Verification items for the finished model (mm, model axes). Face numbers are marked on the shaded views. A direction names the side the tool comes from. Coordinates: 2 decimals unless noted, no trailing zeros. Write each loop counter-clockwise with the first axis right and the second up, starting at its lowest first coordinate (ties: lowest second). Pieces come first, ordered by that corner, then holes. Notation, with made-up numbers: (-30.75, 64.5) - (8.25, 64.5) arc R14 ccw to (8.25, 76.5) - close; hole circle Ø5 at (-4, 14). An arc over 180 degrees is marked (long way). Use one line per item in the form item = value. Start each with the question number.
(1) Gauge pin test, flat ends, axial feed: pin 1 Ø4 at (y, z) = (6.125, -23.275) entering from -X; pin 2 Ø12 at (x, y) = (13.5, 11) entering from +Z; pin 3 Ø3.5 at (x, z) = (5, -25) entering from -Y; pin 4 Ø4 at (x, y) = (-1.5, 22.5) entering from +Z. Record the tip position at first contact, or that the pin passes through.
(2) Material ranges on line 1 (X direction, y = 73.4, z = -38.4); line 2 (X direction, y = 7, z = -18); line 3 (Z direction, x = 11, y = 31), recorded low to high. Write a range as [from, to].
(3) Sectioned sample at D-D (z = -8). Record the cut outline in (x, y).
(4) Sectioned sample at B-B (x = 7). Record the cut outline in (y, z).
(5) Tool access check on the marked faces 1, 2 and 3. Record the directions out of +Z, -Z, +X, -X, +Y, -Y that give a thin tool (end or side, any length) a straight path to the whole face; none if there is none.
(6) Sectioned sample at A-A (z = -38.4). Record the cut outline in (x, y).
(7) Sectioned sample at C-C (y = 29). Record the cut outline in (x, z), and give its area (3 significant figures).
Autodesk Inventor part; units mm, degrees
ref_plane "YZ Plane" through (0, 0, 0) normal (1, 0, 0) x (0, 1, 0)
ref_plane "XZ Plane" through (0, 0, 0) normal (0, 1, 0) x (-1, 0, 0)
ref_plane "XY Plane" through (0, 0, 0) normal (0, 0, 1) x (1, 0, 0)
sketch "Sketch1" plane through (0, 0, 0) normal (0, 1, 0) x (-1, 0, 0)
  line L0 (16.9826, -9.4) -> (-20.8174, -9.4)
  line L1 (-20.8174, -9.4) -> (-20.8174, -29.4)
  line L2 (-20.8174, -29.4) -> (16.9826, -29.4)
  line L3 (16.9826, -29.4) -> (16.9826, -9.4)
  line L4 (7.0826, -29.4) -> (-10.9174, -29.4)
  line L5 (-10.9174, -29.4) -> (-10.9174, -17.15)
  line L6 (-10.9174, -17.15) -> (7.0826, -17.15)
  line L7 (7.0826, -17.15) -> (7.0826, -29.4)
  point P0 (0, 0)
  dimension "d0" = 37.8
  dimension "d1" = 20
  dimension "d2" = 9.9
  dimension "d3" = 9.9
  dimension "d4" = 12.25
extrude "Extrusion1" add sketch "Sketch1" along normal blind 76.05
extrude "Extrusion2" cut sketch "Sketch1" along normal blind 12.25 contours L2 L5 L6 L7
sketch "Sketch2" plane through (0, 0, 0) normal (0, -1, 0) x (1, 0, 0)
  line L0 (-16.9826, -29.4) -> (-16.9826, -9.4)
  line L1 (-16.9826, -9.4) -> (20.8174, -9.4)
  line L2 (20.8174, -9.4) -> (20.8174, 0.6)
  line L3 (20.8174, 0.6) -> (-16.9826, 0.6)
  line L4 (-16.9826, 0.6) -> (-16.9826, -9.4)
  point P0 (0, 0)
  dimension "d10" = 10
extrude "Extrusion3" add sketch "Sketch2" against normal blind 20
sketch "Sketch4" plane through (20.8174, 0, -29.4) normal (1, 0, 0) x (0, 0, -1)
  line L0 (0, 0) -> (-30, 0)
  line L1 (-30, 0) -> (-30, 20)
  line L2 (-30, 0) -> (-30, 20)
  line L3 (-30, 20) -> (-20, 20)
  line L4 (-30, 0) -> (-30, 20)
  line L5 (-20, 20) -> (-30, 0)
  point P0 (-29.4, 0)
  dimension "d14" = 10
extrude "Extrusion4" cut sketch "Sketch4" against normal blind 50
sketch "Sketch5" plane through (20.8174, 76.05, -29.4) normal (0, 0, -1) x (-1, 0, 0)
  line L0 (0, -76.05) -> (0, 0)
  line L1 (37.8, 0) -> (0, 0)
  line L2 (0, 0) -> (0, -5)
  line L3 (0, -5) -> (37.8, -5)
  line L4 (37.8, -5) -> (37.8, 0)
  point P0 (20.8174, -76.05)
  dimension "d17" = 5
extrude "Extrusion5" add sketch "Sketch5" along normal blind 15
fillet "Fillet2" radius 3 1 edges at (1.9174, 71.05, -29.4)
sketch "Sketch6" plane through (-16.9826, 0, -29.4) normal (-1, 0, 0) x (0, 0, 1)
  circle A0 centre (6.125, 6.125) radius 3.125
  line L0 (0, 0) -> (30, 0)
  line L1 (0, 0) -> (0, 68.05)
  point P0 (29.4, 0)
  dimension "d21" = 6.25
  dimension "d22" = 6.125
  dimension "d23" = 6.125
hole "Hole1" at (-16.9826, 6.125, -23.275) direction (1, 0, 0) diameter 6.25 end through all
sketch "Sketch7" plane through (-16.9826, 71.05, -44.4) normal (0, -1, 0) x (1, 0, 0)
  circle A0 centre (10, 6) radius 2.75
  circle A1 centre (27.8, 6) radius 2.75
  line L0 (0, 12) -> (0, 0)
  line L1 (37.8, 12) -> (37.8, 0)
  line L2 (37.8, 0) -> (0, 0)
  line L3 (0, 12) -> (37.8, 12)
  point P0 (16.9826, 44.4)
  point P1 (37.8, 6)
  dimension "d32" = 5.5
  dimension "d33" = 5.5
  dimension "d34" = 10
  dimension "d35" = 10
  dimension "d36" = 6
  dimension "d37" = 6
  dimension "d38" = 6
hole "Hole2" at (-6.9826, 71.05, -38.4) at (10.8174, 71.05, -38.4) direction (0, 1, 0) diameter 3.5 end through all
properties part number "legsv1"
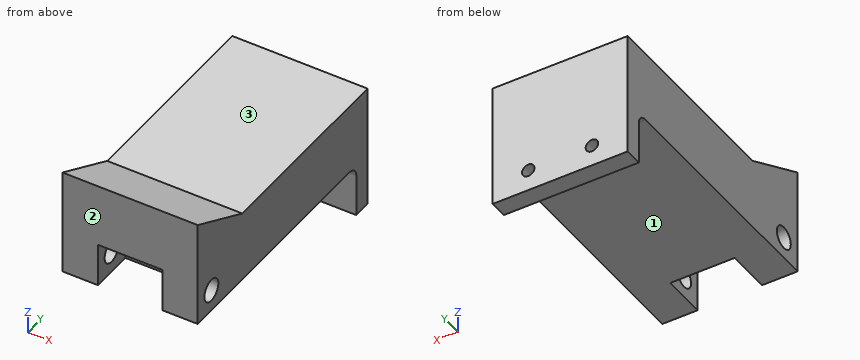
Answers below:
q1.pin_1 = through
q1.pin_2 = -1.9
q1.pin_3 = 12.25
q1.pin_4 = -9.4
q2.line_1 = [-16.98, -8.73], [-5.23, 9.07], [12.57, 20.82]
q2.line_2 = [-16.98, -7.08], [10.92, 20.82]
q2.line_3 = [-29.4, -9.4]
q3.outline = (-16.98, 0) - (20.82, 0) - (20.82, 17.2) - (-16.98, 17.2) - close
q4.outline = (0, -17.15) - (12.25, -17.15) - (12.25, -29.4) - (68.05, -29.4) arc R3 cw to (71.05, -32.4) - (71.05, -44.4) - (76.05, -44.4) - (76.05, -9.4) - (20, -9.4) - (0, 0.6) - close
q5.face_1 = -Z, +X, -X, -Y
q5.face_2 = +Z, -Z, +X, -X, -Y
q5.face_3 = +Z, +X, -X, +Y
q6.outline = (-16.98, 71.05) - (-8.73, 71.05) - (-8.73, 76.05) - (-16.98, 76.05) - close; (-5.23, 71.05) - (9.07, 71.05) - (9.07, 76.05) - (-5.23, 76.05) - close; (12.57, 71.05) - (20.82, 71.05) - (20.82, 76.05) - (12.57, 76.05) - close
q7.outline = (-16.98, -29.4) - (20.82, -29.4) - (20.82, -9.4) - (-16.98, -9.4) - close
q7.area = 756 mm2
